from build123d import *

# Parameters (mm, degrees)
SKETCH2_R          = 1.7272
CUT_EXTRUDE1_DEPTH = 7.35


with BuildPart() as part:
    # Sketch1 → Revolve1 (revolve)
    with BuildSketch(Plane.XY, mode=Mode.PRIVATE) as revolve1_sk:
        with BuildLine():
            Line((3, 3.9878), (3, 12.954))
            Line((3, 12.954), (0, 14.686050808))
            Line((0, 14.686050808), (0, 15.875))
            Line((0, 15.875), (5.08, 15.875))
            ThreePointArc((5.08, 15.875), (5.978025612, 15.503025612), (6.35, 14.605))
            Line((6.35, 14.605), (6.35, 3.495842105))
            Line((6.35, 3.495842105), (5.6515, 2.54))
            Line((5.6515, 2.54), (5.6515, 0))
            Line((5.6515, 0), (4.7625, 0))
            Line((4.7625, 0), (4.7625, 3.9878))
            Line((4.7625, 3.9878), (3, 3.9878))
        make_face()
    revolve(revolve1_sk.sketch.rotate(Axis((0, 0, 0), (0, 1, 0)), 90), axis=Axis((0, 0, 0), (0, 1, 0)))  # turned: the seam where the file's is

    # Sketch2 → Cut-Extrude1 (cut, through all)
    with BuildSketch(Plane.XY):
        with Locations(Location((0, 7.239, 0), (0, 0, 90))):  # turned: the seam where the file's is
            Circle(SKETCH2_R)
    extrude(amount=-CUT_EXTRUDE1_DEPTH, mode=Mode.SUBTRACT)


solid = part.part
Input: part model. Units: mm. Frame: model coordinates. A direction names the side the tool comes from. Round coordinates to 2 decimals unless told otherwise and drop trailing zeros. Order: outer loops, then holes, each group sorted by start corner. A loop starts at its lowest first (then second) coordinate and runs counter-clockwise, first axis right, second up. Notation, with made-up numbers: (21.5, 50) - (69.5, 50) arc R21 cw to (69.5, 67) - close; hole circle Ø5 at (51.5, -34). An arc over 180 degrees is marked (long way). Answer as a JSON object with one key per item and string values. Group by question number.
(1) Pin query (flat end, axial travel): P1, Ø2, axis at x = -5, y = 10.5, coming from the -Z side; P2, Ø7.5, axis at x = 0, z = 0, coming from the -Y side; P3, Ø1, axis at y = 5, z = -1, coming from the +X side; P4, Ø4.5, axis at x = 0, y = 7.239, coming from the -Z side. Return the tip coordinate at first contact, or that it passes through.
(2) Reachability of faces 1 (the face through (3, 3.988, -1)), 2 (the face through (4, 0, 3)), 3 (the face through (0.662, 8.834, -4.374)) from +Z, -Z, +X, -X, +Y, -Y: full face, straight path, thin tool, end or side. Return the list, or none.
(3) Cut plane A-A (y = 13.75). Return loops of the section in (x, z), then the cut area to 3 significant figures.
(4) Draft query along X for faces 4 (the face through (5.517, 1.252, 1.225)), 5 (the face through (4.65, 2.02, 1.03)), 6 (the face through (0, 15.875, 0)), 7 (the face through (0, 9, 3)). Return one class per face: released by +X, released by -X, zero draft, split by the parting line, or undercut.
(5) Material intervals for probe 1 along X at (y, z) = (11, 0); probe 2 along X at (y, z) = (1.7, 0); probe 3 along Z at (x, y) = (0.25, 5.25), sorted ascending. Write a range as from..to.
Here are the results:
{
 "1": {"P1": "stops at z = -4.93", "P2": "stops at y = 3.99", "P3": "stops at x = 6.33", "P4": "stops at z = -6.35"},
 "2": {"face 1": "-Y", "face 2": "+Z, -Z, +X, -X, -Y", "face 3": "-Z"},
 "3": {"outline": "circle Ø12.7 at (0, 0); hole circle Ø3.24 at (0, 0)", "area": "118 mm^2"},
 "4": {"face 4": "split by the parting line", "face 5": "undercut", "face 6": "zero draft", "face 7": "undercut"},
 "5": {"probe 1": "x = -6.35..-3, 3..6.35", "probe 2": "x = -5.65..-4.76, 4.76..5.65", "probe 3": "z = -6.35..-2.99, 2.99..6.35"}
}
